Build history of the part. All positions in model axes, mm. A direction names the side the tool comes from. Coordinates: 2 decimals unless noted, no trailing zeros. Order: outer loops, then holes, each group sorted by start corner. A loop starts at its lowest first (then second) coordinate and runs counter-clockwise, first axis right, second up. Notation, with made-up numbers: (-23, 18) -> (-2, 18) arc R17 cw to (-2, 42) -> close; hole circle Ø9 at (10, -1.75). An arc over 180 degrees is marked (long way). Write each question's results on one line, items separated by ' | '.
from build123d import *

# Parameters (mm, degrees)
SKETCH1_W               = 62.865
SKETCH1_H               = 71.12
BOSS_EXTRUDE1_DEPTH     = 7.62
SKETCH2_W               = 35.433
SKETCH2_H               = 43.688
BOSS_EXTRUDE2_DEPTH     = 3.81
SKETCH3_W               = 35.433
SKETCH3_H               = 43.688
CUT_EXTRUDE1_DEPTH      = 3.175
CUT_EXTRUDE2_DEPTH      = 49.068493384
CUT_EXTRUDE2_DEPTH_BACK = 49.068493384
SKETCH4_R               = 3.175


with BuildPart() as part:
    # Sketch1 → Boss-Extrude1 (new body)
    with BuildSketch(Plane.XY):
        Rectangle(SKETCH1_W, SKETCH1_H)
    extrude(amount=BOSS_EXTRUDE1_DEPTH)

    # Sketch2 → Boss-Extrude2 (add)
    with BuildSketch(Plane.XY.offset(7.62)):
        Rectangle(SKETCH2_W, SKETCH2_H)
    extrude(amount=BOSS_EXTRUDE2_DEPTH)

    # Sketch3 → Cut-Extrude1 (cut)
    with BuildSketch(Plane(origin=(0, 0, 0), x_dir=(-1, 0, 0), z_dir=(0, 0, -1))):
        Rectangle(SKETCH3_W, SKETCH3_H)
    extrude(amount=-CUT_EXTRUDE1_DEPTH, mode=Mode.SUBTRACT)

    # Sketch4 → Cut-Extrude2 (cut, two sides: drawn at the far end of the back side and taken through both)
    with BuildSketch(Plane.XY.offset(7.62).offset(-CUT_EXTRUDE2_DEPTH_BACK)):
        with Locations((-12.7, 29.21)):
            Circle(SKETCH4_R)
        with Locations((-25.4, 15.875)):
            Circle(SKETCH4_R)
        with Locations((-12.7, -29.21)):
            Circle(SKETCH4_R)
        with Locations((-25.4, -15.875)):
            Circle(SKETCH4_R)
        with Locations((12.7, -29.21)):
            Circle(SKETCH4_R)
        with Locations((12.7, 29.21)):
            Circle(SKETCH4_R)
        with Locations((25.4, 0)):
            Circle(SKETCH4_R)
        with Locations((25.4, 22.225)):
            Circle(SKETCH4_R)
        with Locations((25.4, -22.225)):
            Circle(SKETCH4_R)
    extrude(amount=CUT_EXTRUDE2_DEPTH + CUT_EXTRUDE2_DEPTH_BACK, mode=Mode.SUBTRACT)


solid = part.part
Item 1: Tool access for faces 4 (the flat face through (0, -21.844, 2)), 5 (the flat face through (0, -21.844, 9)), 6 (the flat face through (17.716, 0, 9)), 7 (the flat face through (-17.716, 0, 9)): list every direction of +Z, -Z, +X, -X, +Y, -Y with a clear straight run to the whole face (end or side of a thin tool).
Answer:
face 4: -Z | face 5: +Z, +X, -X, -Y | face 6: +Z, +X, +Y, -Y | face 7: +Z, -X, +Y, -Y
Item 2: Slice it at C-C, the plane x = 25.4. List the corners of the cut face in (y, z) (3 decimals), and give its area (3 significant figures).
Answer:
outline: (-35.56, 0) -> (-25.4, 0) -> (-25.4, 7.62) -> (-35.56, 7.62) -> close; (-19.05, 0) -> (-3.175, 0) -> (-3.175, 7.62) -> (-19.05, 7.62) -> close; (3.175, 0) -> (19.05, 0) -> (19.05, 7.62) -> (3.175, 7.62) -> close; (25.4, 0) -> (35.56, 0) -> (35.56, 7.62) -> (25.4, 7.62) -> close | area: 397 mm^2
Item 3: Slice it at A-A, the plane x = -25.4. List the corners of the cut face in (y, z), and give its area (3 significant figures).
Answer:
outline: (-35.56, 0) -> (-19.05, 0) -> (-19.05, 7.62) -> (-35.56, 7.62) -> close; (-12.7, 0) -> (12.7, 0) -> (12.7, 7.62) -> (-12.7, 7.62) -> close; (19.05, 0) -> (35.56, 0) -> (35.56, 7.62) -> (19.05, 7.62) -> close | area: 445 mm^2
Item 4: Slice it at B-B, the plane y = 29.21. List the corners of the cut face in (x, z) (1 decimal).
Answer:
outline: (-31.4, 0) -> (-15.9, 0) -> (-15.9, 7.6) -> (-31.4, 7.6) -> close; (-9.5, 0) -> (9.5, 0) -> (9.5, 7.6) -> (-9.5, 7.6) -> close; (15.9, 0) -> (31.4, 0) -> (31.4, 7.6) -> (15.9, 7.6) -> close
Item 5: Pull direction Y, two halves, no side cores. Call faces 1 (the flat face through (0, 21.844, 2)), 2 (the flat face through (0, -35.56, 4)), 3 (the flat face through (0, 21.844, 9)): released by +Y, released by -Y, zero draft, split by the parting line, or undercut.
Answer:
face 1: undercut | face 2: released by -Y | face 3: released by +Y
Item 6: Slice it at D-D, the plane z = 4.75. State how many separate pieces and enclosed holes the cut face has, and give its area (3 significant figures).
Answer:
separate pieces: 1 | enclosed holes: 9 | area: 4,190 mm^2
Item 7: Drill centre lines: line 1 (Y direction, x = 25.4, z = 3.75) (3 decimals); line 2 (Y direction, x = 12.7, z = 2.25) (3 decimals); line 3 (X direction, y = 29.21, z = 6) (1 decimal). Where is each one in solid material? Low to high. Write a range as from..to.
Answer:
line 1: y = -35.56..-25.4, -19.05..-3.175, 3.175..19.05, 25.4..35.56 | line 2: y = -35.56..-32.385, -26.035..-21.844, 21.844..26.035, 32.385..35.56 | line 3: x = -31.4..-15.9, -9.5..9.5, 15.9..31.4
Item 8: Pin check, flat tips, straight feed: pin 1 (3 mm diameter, centred on x = -14, y = -5.5, fed in from -Z) (3 decimals); pin 2 (1.1 mm diameter, centred on y = 1.5, z = 9.5, fed in from -X); pin 3 (3 mm diameter, centred on x = 1, z = 10, fed in from +Y). Stop position of each tip, or through.
Answer:
pin 1: stops at z = 3.175 | pin 2: stops at x = -17.72 | pin 3: stops at y = 21.84
